The listing builds one solid part. Answer for the finished solid, in the listing's coordinates (mm). Give positions to 0.01 mm unless a question says otherwise; leave off trailing zeros. Loops run counter-clockwise (first coordinate to the right, second up) from the corner with the lowest first, then second, coordinate; pieces in that order, holes last.
Item 1: Section A-A, the plane z = -10.2 is taken. Give the vertices of the cut face in (x, y), and give its area (3 significant figures).
Item 2: Consider line 1 along X through (y, z) = (-0.75, 10.2); line 2 along X through (y, z) = (-0.5, 11.75). Determine where each line is inside the solid, lowest interval first.
Item 3: Section B-B, the plane x = -5.85 is taken. Give the vertices of the cut face in (y, z).
Item 4: Section C-C, the plane y = -1.6 is taken. Give the vertices of the cut face in (x, z).
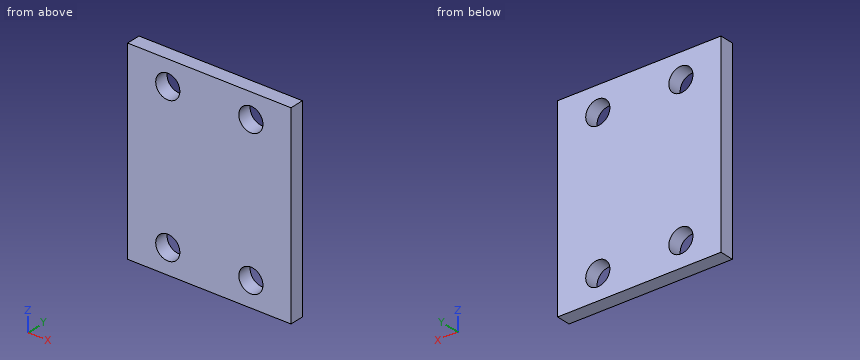
from build123d import *

# Parameters (mm, degrees)
SKETCH1_W           = 23
SKETCH1_H           = 27.4
SKETCH1_R           = 1.7
BOSS_EXTRUDE1_DEPTH = 2


with BuildPart() as part:
    # Sketch1 → Boss-Extrude1 (new body)
    with BuildSketch(Plane(origin=(0, 0, 0), x_dir=(1, 0, 0), z_dir=(0, 1, 0))):
        Rectangle(SKETCH1_W, SKETCH1_H)
        with Locations(Location((5.85, 10.2, 0), (0, 0, 270))):
            Circle(SKETCH1_R, mode=Mode.SUBTRACT)
        with Locations(Location((-5.85, 10.2, 0), (0, 0, 270))):
            Circle(SKETCH1_R, mode=Mode.SUBTRACT)
        with Locations(Location((5.85, -10.2, 0), (0, 0, 270))):
            Circle(SKETCH1_R, mode=Mode.SUBTRACT)
        with Locations(Location((-5.85, -10.2, 0), (0, 0, 270))):
            Circle(SKETCH1_R, mode=Mode.SUBTRACT)
    extrude(amount=-BOSS_EXTRUDE1_DEPTH)


solid = part.part
Worked answers:
1. outline: (-11.5, -2) - (-7.55, -2) - (-7.55, 0) - (-11.5, 0) - close; (-4.15, -2) - (4.15, -2) - (4.15, 0) - (-4.15, 0) - close; (7.55, -2) - (11.5, -2) - (11.5, 0) - (7.55, 0) - close
1. area: 32.4 mm2
2. line 1: x = -11.5 to -7.55, -4.15 to 4.15, 7.55 to 11.5
2. line 2: x = -11.5 to -6.55, -5.15 to 5.15, 6.55 to 11.5
3. outline: (-2, -13.7) - (0, -13.7) - (0, -11.9) - (-2, -11.9) - close; (-2, -8.5) - (0, -8.5) - (0, 8.5) - (-2, 8.5) - close; (-2, 11.9) - (0, 11.9) - (0, 13.7) - (-2, 13.7) - close
4. outline: (-11.5, -13.7) - (11.5, -13.7) - (11.5, 13.7) - (-11.5, 13.7) - close; hole circle Ø3.4 at (-5.85, -10.2); hole circle Ø3.4 at (-5.85, 10.2); hole circle Ø3.4 at (5.85, -10.2); hole circle Ø3.4 at (5.85, 10.2)
